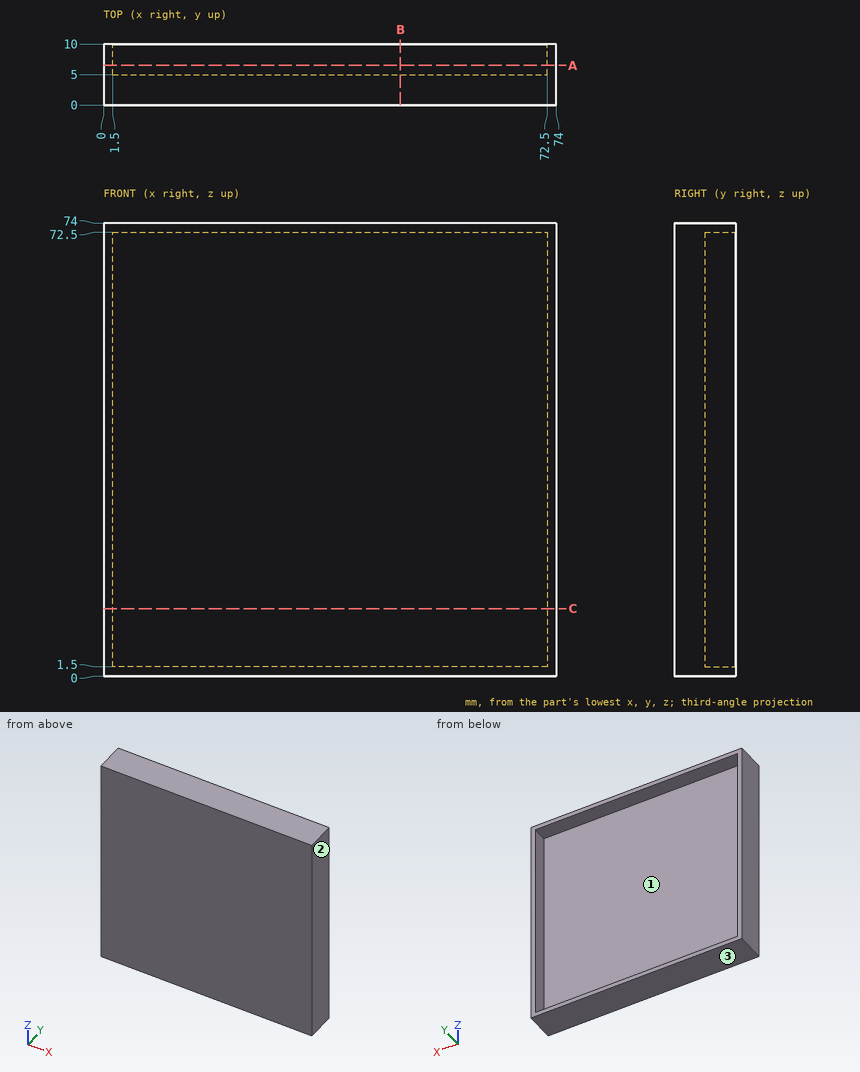
Here's the drawing with two shaded views (mm, measured from the low corner). I have some questions. Coordinates: 2 decimals unless noted, no trailing zeros. Loops run counter-clockwise (first coordinate to the right, second up) from the corner with the lowest first, then second, coordinate; pieces in that order, holes last. Notation, with made-up numbers: M -25.75,70.5 L -0.75,70.5 A28 cw -0.75,105.5 Z; hole C -6.75,87 d2. An arc over 180 degrees is marked long. Return JSON: item names as keys, results as strings. Group by question number.
Item 1: If I drill on L1, parallel to X at y = 9, z = 11; L2, parallel to Y at x = 21.5, z = 67, over which ranges is the centre line in solid material (lowest first)? Write a range as from..to.
Item 2: Thinking about a two-plate mould opening in Z: for the marked faces 1, 2 and 3, which applies, released by +Z, released by -Z, zero draft, split by the parting line, or undercut?
Item 3: Imagine slicing it at B-B (x = 48.5). Please give me the cut outline in (y, z).
Item 4: I'm going to push flat-ended pins straight in: pin 1 Ø5 at (y, z) = (4, 23.5) entering from -X; pin 2 Ø8 at (x, z) = (55, 13) entering from +Y. Where does each tip first touch, or does it pass through?
Item 5: Imagine slicing it at C-C (z = 11). Please give me the cut outline in (x, y), and give its area (3 significant figures).
Item 6: Imagine slicing it at A-A (y = 6.5). Please give me the cut outline in (x, z), and give its area (3 significant figures).
Verdict:
{
 "1": {"L1": "x = 0..1.5, 72.5..74", "L2": "y = 0..5"},
 "2": {"face 1": "undercut", "face 2": "zero draft", "face 3": "released by -Z"},
 "3": {"outline": "M 0,0 L 10,0 L 10,1.5 L 5,1.5 L 5,72.5 L 10,72.5 L 10,74 L 0,74 Z"},
 "4": {"pin 1": "stops at x = 0", "pin 2": "stops at y = 5"},
 "5": {"outline": "M 0,0 L 74,0 L 74,10 L 72.5,10 L 72.5,5 L 1.5,5 L 1.5,10 L 0,10 Z", "area": "385 mm^2"},
 "6": {"outline": "M 0,0 L 74,0 L 74,74 L 0,74 Z; hole M 1.5,1.5 L 72.5,1.5 L 72.5,72.5 L 1.5,72.5 Z", "area": "435 mm^2"}
}
